For this review, use the dimensioned drawing (mm, ordinates from the lowest corner) and the shaded views. Coordinates: 2 decimals unless noted, no trailing zeros. Loops run counter-clockwise (first coordinate to the right, second up) from the corner with the lowest first, then second, coordinate; pieces in that order, holes last. Notation, with made-up numbers: (68.25, -36) - (82.25, -36) arc R27 ccw to (82.25, -6) - close; hole circle Ø2 at (77, -25.5). An arc over 180 degrees is marked (long way). One line per item, written item: value. Start each with the question number.
1. We need section D-D, the plane z = 24. Give the boundary of the cut face in (x, y).
2. To check wall thickness, follow line 1 (X direction, y = 0.65, z = 33); line 2 (Z direction, x = 26.5, y = 2.2); line 3 (X direction, y = 2.7, z = 7). State the ranges of each line that lie inside material, in increasing order.
3. We need section C-C, the plane x = 112. Give the boundary of the cut face in (y, z).
4. We need section A-A, the plane z = 33. Give the boundary of the cut face in (x, y).
5. Insertion check: P1, Ø3, axis at x = 16, z = 33, coming from the -Y side; P2, Ø0.9, axis at y = 1, z = 19.5, coming from the +X side. Each pin has a flat end and moves straight along its axis. Give the tip position at first contact, or say it passes through.
6. We need section B-B, the plane y = 2.55. Give the boundary of the cut face in (x, z).
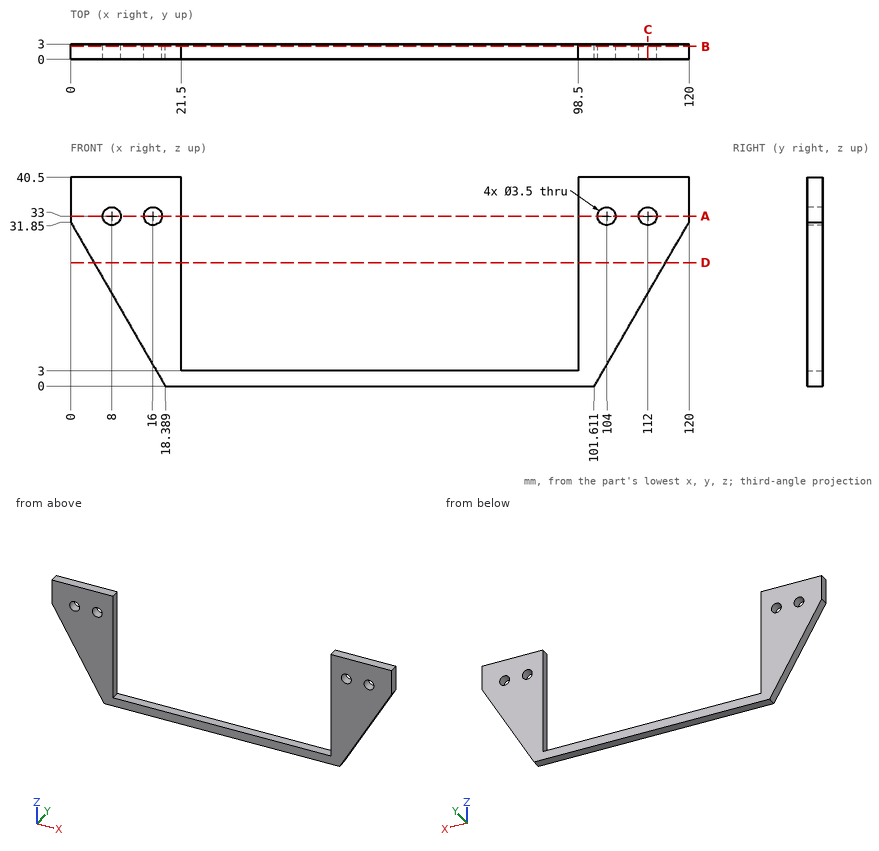
Findings below:
1. outline: (4.53, 0) - (21.5, 0) - (21.5, 3) - (4.53, 3) - close; (98.5, 0) - (115.47, 0) - (115.47, 3) - (98.5, 3) - close
2. line 1: 0 to 6.25, 9.75 to 14.25, 17.75 to 21.5, 98.5 to 102.25, 105.75 to 110.25, 113.75 to 120
2. line 2: 0 to 3
2. line 3: 14.35 to 21.5, 98.5 to 105.65
3. outline: (0, 17.99) - (3, 17.99) - (3, 31.25) - (0, 31.25) - close; (0, 34.75) - (3, 34.75) - (3, 40.5) - (0, 40.5) - close
4. outline: (0, 0) - (6.25, 0) - (6.25, 3) - (0, 3) - close; (9.75, 0) - (14.25, 0) - (14.25, 3) - (9.75, 3) - close; (17.75, 0) - (21.5, 0) - (21.5, 3) - (17.75, 3) - close; (98.5, 0) - (102.25, 0) - (102.25, 3) - (98.5, 3) - close; (105.75, 0) - (110.25, 0) - (110.25, 3) - (105.75, 3) - close; (113.75, 0) - (120, 0) - (120, 3) - (113.75, 3) - close
5. P1: through
5. P2: x = 113.13
6. outline: (0, 31.85) - (18.39, 0) - (101.61, 0) - (120, 31.85) - (120, 40.5) - (98.5, 40.5) - (98.5, 3) - (21.5, 3) - (21.5, 40.5) - (0, 40.5) - close; hole circle Ø3.5 at (8, 33); hole circle Ø3.5 at (16, 33); hole circle Ø3.5 at (104, 33); hole circle Ø3.5 at (112, 33)
